```python
from build123d import *

# Parameters (mm, degrees)
SKETCH1_W                    = 12.7
SKETCH1_H                    = 1.524
BASE_FLANGE1_DEPTH           = 12.7
EDGE_FLANGE2_STRIP_W         = 6.604
EDGE_FLANGE2_STRIP_H         = 1.524
EDGE_FLANGE2_STRIP_CUT_DEPTH = 12.7
EDGE_FLANGE2_DEPTH           = 12.7
EDGE_FLANGE4_STRIP_W         = 6.604
EDGE_FLANGE4_STRIP_H         = 1.524
EDGE_FLANGE4_STRIP_CUT_DEPTH = 12.7
EDGE_FLANGE4_DEPTH           = 12.7


# Sheet-metal steps are written as plain solids
with BuildPart() as part:
    # Sketch1 → Base-Flange1 (new body)
    with BuildSketch(Plane.XY):
        with Locations((6.35, -0.762)):
            Rectangle(SKETCH1_W, SKETCH1_H)
    extrude(amount=BASE_FLANGE1_DEPTH)

    # Edge-Flange2 strip (across the edge) → Edge-Flange2 strip cut (cut)
    with BuildSketch(Plane(origin=(0, 0, 12.7), x_dir=(0, 0, -1), z_dir=(1, 0, 0))):
        with Locations((-3.048, -0.762)):
            Rectangle(EDGE_FLANGE2_STRIP_W, EDGE_FLANGE2_STRIP_H)
    extrude(amount=EDGE_FLANGE2_STRIP_CUT_DEPTH, mode=Mode.SUBTRACT)

    # Edge-Flange2 section (across the edge) → Edge-Flange2 (add)
    with BuildSketch(Plane(origin=(0, 0, 12.7), x_dir=(0, 0, -1), z_dir=(1, 0, 0))):
        with BuildLine():
            Line((-1.524, 0.254), (-1.524, 4.276))
            Line((-1.524, 4.276), (0, 4.276))
            Line((0, 4.276), (0, 0.254))
            ThreePointArc((0, 0.254), (0.074394878, 0.074394878), (0.254, 0))
            Line((0.254, 0), (0.254, -1.524))
            ThreePointArc((0.254, -1.524), (-1.003235857, -1.003235857), (-1.524, 0.254))
        make_face()
    extrude(amount=EDGE_FLANGE2_DEPTH)

    # Sketch10 → CSK for M3 SFHCS1 (revolve, cut)
    with BuildSketch(Plane(origin=(6.35, 0, 6.35), x_dir=(0, 0, 1), z_dir=(1, 0, 0))):
        Polygon((0, 0), (0, 1.524), (1.7, 1.524), (1.7, 1.66), (3.36, 0), align=None)
    revolve(axis=Axis((6.35, 6.35, 6.35), (0, -1, 0)), mode=Mode.SUBTRACT)

    # Edge-Flange4 strip (across the edge) → Edge-Flange4 strip cut (cut)
    with BuildSketch(Plane(origin=(12.7, 4.276, 14.224), x_dir=(0, -1, 0), z_dir=(-1, 0, 0))):
        with Locations((-1.524, -0.762)):
            Rectangle(EDGE_FLANGE4_STRIP_W, EDGE_FLANGE4_STRIP_H)
    extrude(amount=EDGE_FLANGE4_STRIP_CUT_DEPTH, mode=Mode.SUBTRACT)

    # Edge-Flange4 section (across the edge) → Edge-Flange4 (add)
    with BuildSketch(Plane(origin=(12.7, 4.276, 14.224), x_dir=(0, -1, 0), z_dir=(-1, 0, 0))):
        with BuildLine():
            Line((0, 0.254), (0, 11.176))
            Line((0, 11.176), (1.524, 11.176))
            Line((1.524, 11.176), (1.524, 0.254))
            ThreePointArc((1.524, 0.254), (1.598394878, 0.074394878), (1.778, 0))
            Line((1.778, 0), (1.778, -1.524))
            ThreePointArc((1.778, -1.524), (0.520764143, -1.003235857), (0, 0.254))
        make_face()
    extrude(amount=EDGE_FLANGE4_DEPTH)


solid = part.part
```
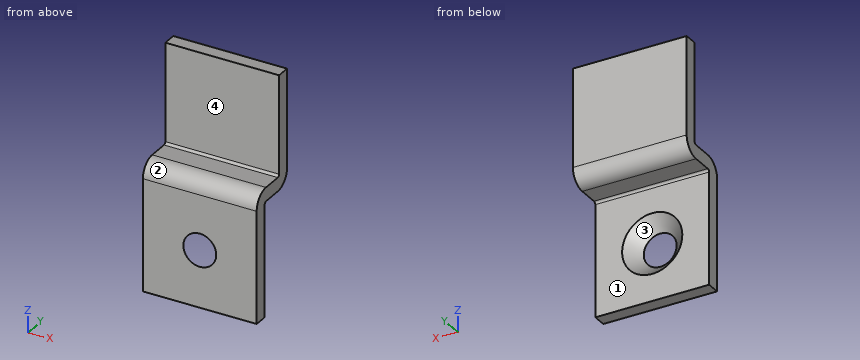
CAD build for the part. Positions are in the model's coordinates, mm. Face numbers are marked on the shaded views. A direction names the side the tool comes from. Coordinates: 2 decimals unless noted, no trailing zeros. Order: outer loops, then holes, each group sorted by start corner. A loop starts at its lowest first (then second) coordinate and runs counter-clockwise, first axis right, second up. Notation, with made-up numbers: (63.25, -26.75) - (81.25, -26.75) arc R26 ccw to (81.25, -0.75) - close; hole circle Ø11 at (-1.75, 11). An arc over 180 degrees is marked (long way). Answer in a Markdown table with one row per item.
1. Pull direction X, two halves, no side cores. Call the marked faces 3 and 4: +X half, -X half, draft (parallel to the pull), parting line (faces both ways), or undercut.
Answer:
| item | result |
|---|---|
| face 3 | undercut |
| face 4 | draft |
2. Drill centre lines: L1, parallel to Y at x = 1, z = 14.75; L2, parallel to Z at x = 3.25, y = 0.6; L3, parallel to Y at x = 10, z = 7.75. Where is each one in solid material? Low to high. Write a range as from..to.
Answer:
| item | result |
|---|---|
| L1 | 2.75..4.28 |
| L2 | 12.7..14.22 |
| L3 | -1.52..0 |
3. 3-axis set-ups, long thin cutter, end or side, ignore diameter. For the marked faces 1 and 2: which of +Z, -Z, +X, -X, +Y, -Y reach the whole face in a straight line?
Answer:
| item | result |
|---|---|
| face 1 | -Z, +X, -X, +Y |
| face 2 | +Z, +X, -X, -Y |
4. Slice it at B-B, the plane z = 6.35. List the corners of the cut face in (x, y).
Answer:
| item | result |
|---|---|
| outline | (0, -1.52) - (4.51, -1.52) - (2.99, 0) - (0, 0) - close; (8.19, -1.52) - (12.7, -1.52) - (12.7, 0) - (9.71, 0) - close |
5. Slice it at D-D, the plane z = 20.75. List the corners of the cut face in (x, y).
Answer:
| item | result |
|---|---|
| outline | (0, 2.75) - (12.7, 2.75) - (12.7, 4.28) - (0, 4.28) - close |
6. Slice it at C-C, the plane x = 6.35. List the corners of the cut face in (y, z).
Answer:
| item | result |
|---|---|
| outline | (-1.52, 0) - (0, 0) - (0, 2.99) - (-1.52, 4.51) - close; (-1.52, 8.19) - (0, 9.71) - (0, 12.45) arc R0.25 cw to (0.25, 12.7) - (2.5, 12.7) arc R1.78 ccw to (4.28, 14.48) - (4.28, 25.4) - (2.75, 25.4) - (2.75, 14.48) arc R0.25 cw to (2.5, 14.22) - (0.25, 14.22) arc R1.78 ccw to (-1.52, 12.45) - close |
7. Flat gauge pins, fed straight in: P1, Ø1.1, axis at x = 5.5, y = 1.5, coming from the +Z side; P2, Ø2.5, axis at x = 7.5, y = 2, coming from the -Z side; P3, Ø6, axis at x = 4.5, z = 3.5, coming from the +Y side. Where does each tip first touch, or does it go through?
Answer:
| item | result |
|---|---|
| P1 | z = 14.22 |
| P2 | z = 12.7 |
| P3 | y = 0 |
8. Slice it at A-A, the plane x = 10.5. List the corners of the cut face in (y, z), then the cut area to 3 significant figures.
Answer:
| item | result |
|---|---|
| outline | (-1.52, 0) - (0, 0) - (0, 12.45) arc R0.25 cw to (0.25, 12.7) - (2.5, 12.7) arc R1.78 ccw to (4.28, 14.48) - (4.28, 25.4) - (2.75, 25.4) - (2.75, 14.48) arc R0.25 cw to (2.5, 14.22) - (0.25, 14.22) arc R1.78 ccw to (-1.52, 12.45) - close |
| area | 43.9 mm² |
